Can you work these out from the model? Positions are in its coordinate system, mm. A direction names the side the tool comes from. Coordinates: 2 decimals unless noted, no trailing zeros. Order: outer loops, then holes, each group sorted by start corner. A loop starts at its lowest first (then second) coordinate and runs counter-clockwise, first axis right, second up. Notation, with made-up numbers: (-28.5, 48) - (13.5, 48) arc R15 ccw to (13.5, 60) - close; hole circle Ø1 at (55.5, 53.25). An arc over 180 degrees is marked (long way). Return JSON: item names as keys, results as strings. Group by question number.
1) If we mould it in two halves opening along Z, with no side actions, what happens to faces 6 (the face through (-42.6, 12.3, 1)), 7 (the face through (-26, 0, 2)), 8 (the face through (27.7, -8, 10.5))? For each: pulls with the +Z half, pulls with the -Z half, needs draft (parallel to the pull), parting line crosses it, or undercut.
2) Imagine slicing it at A-A (y = -9). Write out the boundary of the cut face in (x, z).
3) Which directions (+Z, -Z, +X, -X, +Y, -Y) give clear straight access to the entire face, cutting with the end or side of a thin tool? Please do faces 1 (the face through (13.517, -17, 3)), 2 (the face through (14, 5, 2)), 3 (the face through (21, -4.75, 21)), 4 (the face through (26.437, -0.308, 10.117)), 5 (the face through (-18.1, -12.3, 1)).
4) Imagine slicing it at C-C (x = -14). Write out the boundary of the cut face in (y, z).
5) Imagine slicing it at D-D (z = 5.75). Write out the boundary of the cut face in (x, y), and give its area (3 significant figures).
6) If I drill on line 1 along Z through (x, y) = (20, 3); line 2 along Z through (x, y) = (-35, -5); line 3 along Y through (x, z) = (23.5, 20.5), over which ranges is the centre line in solid material (lowest first)?
7) Imagine slicing it at B-B (y = -4). Write out the boundary of the cut face in (x, z), and give its area (3 significant figures).
8) For pin 1 Ø4 at (x, y) = (-39.5, 16) entering from -Z; pin 2 Ø12 at (y, z) = (12.5, 16.5) entering from -X; pin 3 Ø7 at (x, y) = (9, 6.5) entering from -Z; pin 4 Ø22 at (x, y) = (-16, 0) entering from +Z, each with a flat end and sliding along its axis, tell me the tip position at first contact or that it passes through.
```python
from build123d import *

# Parameters (mm, degrees)
F1_DEPTH  = 22
F3_DEPTH  = 2
F5_DEPTH  = 25
F7_DEPTH  = 25
F9_DEPTH  = 2
F11_DEPTH = 2.4954547296
F13_DEPTH = 2
F14_DEPTH = 25


# Not quite as in the source:
# - a feature names something its author has since deleted; it is built from what else it names


with BuildPart() as f1:
    # F0 (on Front) → F1 (new body, symmetric)
    with BuildSketch(Plane.XZ):
        with BuildLine():
            Line((-40, 0), (-0.4058661959, 0))
            ThreePointArc((-0.4058661959, 0), (-0.0297944203, 0.073409465), (0.2910628996, 0.2828599608))
            Line((0.2910628996, 0.2828599608), (1.7669371004, 1.7171400392))
            ThreePointArc((1.7669371004, 1.7171400392), (2.0877944203, 1.926590535), (2.4638661959, 2))
            Line((2.4638661959, 2), (26.037, 2))
            ThreePointArc((26.037, 2), (27.9687843496, 2.7891547709), (28.7954749436, 4.705176349))
            Line((28.7954749436, 4.705176349), (29.016465998, 16.0310205539))
            ThreePointArc((29.016465998, 16.0310205539), (28.8276722638, 16.8546583092), (28.2736767263, 17.4927109486))
            Line((28.2736767263, 17.4927109486), (27.3333525812, 18.1512658075))
            Line((27.3333525812, 18.1512658075), (26.1860444646, 16.5130704329))
            Line((26.1860444646, 16.5130704329), (26.8254471929, 16.0652655182))
            Line((26.8254471929, 16.0652655182), (26.037, 4))
            Line((26.037, 4), (1.4428661959, 4))
            ThreePointArc((1.4428661959, 4), (1.0667944203, 3.926590535), (0.7459371004, 3.7171400392))
            Line((0.7459371004, 3.7171400392), (-0.7299371004, 2.2828599608))
            ThreePointArc((-0.7299371004, 2.2828599608), (-1.0507944203, 2.073409465), (-1.4268661959, 2))
            Line((-1.4268661959, 2), (-40, 2))
            Line((-40, 2), (-40, 0))
        make_face()
    extrude(amount=F1_DEPTH, both=True)

    # F2 (on face) → F3 (join)
    with BuildSketch(Plane.XY.offset(2)):
        with BuildLine():
            Line((-50, 12), (-50, -12))
            ThreePointArc((-50, -12), (-47.0710678119, -19.0710678119), (-40, -22))
            Line((-40, -22), (-40, 22))
            ThreePointArc((-40, 22), (-47.0710678119, 19.0710678119), (-50, 12))
        make_face()
    extrude(amount=-F3_DEPTH)

    # F4 (on face) → F5 (cut)
    with BuildSketch(Plane.XY.offset(2)):
        with BuildLine():
            ThreePointArc((-40.35, 14.489), (-42.6, 12.239), (-40.35, 9.989))
            Line((-40.35, 9.989), (-20.35, 9.989))
            ThreePointArc((-20.35, 9.989), (-18.1, 12.239), (-20.35, 14.489))
            Line((-20.35, 14.489), (-40.35, 14.489))
        make_face()
    extrude(amount=-F5_DEPTH, mode=Mode.SUBTRACT)

    # F6 (on face) → F7 (cut)
    with BuildSketch(Plane(origin=(28.6927430868, 0, -0.5598557981), x_dir=(0, 1, 0), z_dir=(0.9998096932, 0, -0.0195083911))):
        with BuildLine():
            Line((-9.9999997095, 13.096034309), (-17.9999997095, 13.096034309))
            ThreePointArc((-17.9999997095, 13.096034309), (-20, 11.0960344543), (-18, 9.096034309))
            Line((-18, 9.096034309), (-9.9999997095, 9.096034309))
            ThreePointArc((-9.9999997095, 9.096034309), (-7.9999997095, 11.096034309), (-9.9999997095, 13.096034309))
        make_face()
    extrude(amount=-F7_DEPTH, mode=Mode.SUBTRACT)

    # F8 (on face) → F9 (join)
    with BuildSketch(Plane(origin=(17.5237251574, 0, 25.0214263138), x_dir=(0.8190976873, 0, -0.5736540583), z_dir=(0.5736540583, 0, 0.8190976873))):
        with BuildLine():
            Line((2.9761385921, 13), (2.9761385921, -13))
            ThreePointArc((2.9761385921, -13), (5.6121775614, -19.3639610307), (11.9761385921, -22))
            Line((11.9761385921, -22), (11.9761385921, 22))
            ThreePointArc((11.9761385921, 22), (5.6121775614, 19.3639610307), (2.9761385921, 13))
        make_face()
    extrude(amount=-F9_DEPTH)

    # F10 (on face) → F11 (cut, through all)
    with BuildSketch(Plane(origin=(17.5237251574, 0, 25.0214263138), x_dir=(0.8190976873, 0, -0.5736540583), z_dir=(0.5736540583, 0, 0.8190976873))):
        with BuildLine():
            Line((2.9761385921, 4.75), (2.9761385921, -4.75))
            Line((2.9761385921, -4.75), (7.9761385921, -4.75))
            ThreePointArc((7.9761385921, -4.75), (13.0569949576, 0), (7.9761385921, 4.75))
            Line((7.9761385921, 4.75), (2.9761385921, 4.75))
        make_face()
    extrude(amount=-F11_DEPTH, mode=Mode.SUBTRACT)

    # F12 (on face) → F13 (cut, through all)
    with BuildSketch(Plane(origin=(0, 0, 2), x_dir=(1, 0, 0), z_dir=(0, 0, -1))):
        with BuildLine():
            Line((22.517, 12), (22.517, 22))
            Line((22.517, 22), (13.517, 22))
            Line((13.517, 22), (13.517, 12))
            ThreePointArc((13.517, 12), (18.017, 7.5), (22.517, 12))
        make_face()
    extrude(amount=-F13_DEPTH, mode=Mode.SUBTRACT)

    # F4 (on face) → F14 (cut)
    with BuildSketch(Plane.XY.offset(2)):
        with BuildLine():
            Line((-20.35, -9.989), (-40.35, -9.989))
            ThreePointArc((-40.35, -9.989), (-42.6, -12.239), (-40.35, -14.489))
            Line((-40.35, -14.489), (-20.35, -14.489))
            ThreePointArc((-20.35, -14.489), (-18.1, -12.239), (-20.35, -9.989))
        make_face()
    extrude(amount=-F14_DEPTH, mode=Mode.SUBTRACT)


solid = f1.part
```
Calculated:
{
 "1": {"face 6": "needs draft", "face 7": "pulls with the +Z half", "face 8": "undercut"},
 "2": {"outline": "(-50, 0) - (-0.41, 0) arc R1 ccw to (0.29, 0.28) - (1.77, 1.72) arc R1 cw to (2.46, 2) - (14.66, 2) - (14.66, 4) - (1.44, 4) arc R1 ccw to (0.75, 3.72) - (-0.73, 2.28) arc R1 cw to (-1.43, 2) - (-50, 2) - close; (18.81, 21.68) - (26.83, 16.07) - (26.58, 12.31) - (28.94, 12.27) - (29.02, 16.03) arc R1.74 ccw to (28.27, 17.49) - (19.96, 23.31) - close; (21.37, 2) - (26.04, 2) arc R2.76 ccw to (28.8, 4.71) - (28.88, 8.8) - (26.35, 8.85) - (26.04, 4) - (21.37, 4) - close"},
 "3": {"face 1": "+Z, -Z, -Y", "face 2": "-Z, +X, +Y, -Y", "face 3": "+Z, -X", "face 4": "-X, +Y, -Y", "face 5": "+Z, -Z"},
 "4": {"outline": "(-22, 0) - (22, 0) - (22, 2) - (-22, 2) - close"},
 "5": {"outline": "(26.15, -22) - (28.82, -22) - (28.82, 22) - (26.15, 22) - close", "area": "117 mm2"},
 "6": {"line 1": "2 to 4", "line 2": "0 to 2", "line 3": "-20.8 to -4.75, 4.75 to 20.8"},
 "7": {"outline": "(-50, 0) - (-0.41, 0) arc R1 ccw to (0.29, 0.28) - (1.77, 1.72) arc R1 cw to (2.46, 2) - (26.04, 2) arc R2.76 ccw to (28.8, 4.71) - (29.02, 16.03) arc R1.74 ccw to (28.27, 17.49) - (26.43, 18.78) - (25.29, 17.14) - (26.83, 16.07) - (26.04, 4) - (1.44, 4) arc R1 ccw to (0.75, 3.72) - (-0.73, 2.28) arc R1 cw to (-1.43, 2) - (-50, 2) - close", "area": "194 mm2"},
 "8": {"pin 1": "z = 0", "pin 2": "x = 18.81", "pin 3": "z = 2", "pin 4": "z = 2"}
}
